```python
from build123d import *

# Parameters (mm, degrees)
F1_DEPTH = 12.7


with BuildPart() as f1:
    # F0 (on Front) → F1 (new body, symmetric)
    with BuildSketch(Plane.XZ):
        Polygon((-41.637809, 68.136583), (-89.650807, -58.443111), (-62.147316, -58.70938), (-31.672317, 17.590671), (0, -58.70938), (90.179723, -58.70938), (75.366612, -24.786401), (48.944038, -24.786401), (52.657543, -33.30938), (15.323475, -33.30938), (-17.810837, 42.736583), (23.85487, 42.736583), (27.09148, 35.308142), (54.189362, 35.308142), (41.60433, 68.136583), align=None)
    extrude(amount=F1_DEPTH, both=True)


solid = f1.part
```
Verification items for the finished model (mm, model axes). A direction names the side the tool comes from. Coordinates: 2 decimals unless noted, no trailing zeros. Loops run counter-clockwise (first coordinate to the right, second up) from the corner with the lowest first, then second, coordinate; pieces in that order, holes last. Notation, with made-up numbers: (72, 15.25) - (114, 15.25) arc R15 cw to (114, 36.25) - close; hole circle Ø10 at (-2.75, 0). An arc over 180 degrees is marked (long way). Return JSON: item names as keys, results as strings.
1. Section check B-B, the plane y = -7. Record the boundary of the cut face in (x, z), then the cut area to 3 significant figures.
Established:
{"outline": "(-89.65, -58.44) - (-62.15, -58.71) - (-31.67, 17.59) - (0, -58.71) - (90.18, -58.71) - (75.37, -24.79) - (48.94, -24.79) - (52.66, -33.31) - (15.32, -33.31) - (-17.81, 42.74) - (23.85, 42.74) - (27.09, 35.31) - (54.19, 35.31) - (41.6, 68.14) - (-41.64, 68.14) - close", "area": "9,620 mm2"}
2. Section check D-D, the plane x = -59. Record the boundary of the cut face in (y, z), then the cut area to 3 significant figures.
Established:
{"outline": "(-12.7, -50.83) - (12.7, -50.83) - (12.7, 22.36) - (-12.7, 22.36) - close", "area": "1,860 mm2"}
3. Mould release check, pull along X, two halves, no side actions. Record for faces 1 (the flat face through (-65.31, -0.18, 5.73)), 2 (the flat face through (-16.058, -0.178, -20.025)), 3 (the flat face through (-1, 12.7, -8)): +X half, -X half, draft (parallel to the pull), parting line (faces both ways), or undercut.
Established:
{"face 1": "-X half", "face 2": "undercut", "face 3": "draft"}
4. Tool access check on faces 4 (the flat face through (50.775, -0.178, -28.988)), 5 (the flat face through (-47.12, -0.18, -21.09)), 6 (the flat face through (62, 0, -24.786)), 7 (the flat face through (1, 0, 68.137)). Record the directions out of +Z, -Z, +X, -X, +Y, -Y that give a thin tool (end or side, any length) a straight path to the whole face; none if there is none.
Established:
{"face 4": "+Y, -Y", "face 5": "-Z, +Y, -Y", "face 6": "+X, +Y, -Y", "face 7": "+Z, +X, -X, +Y, -Y"}
5. Section check C-C, the plane z = 3. Record the boundary of the cut face in (x, y).
Established:
{"outline": "(-66.34, -12.7) - (-37.5, -12.7) - (-37.5, 12.7) - (-66.34, 12.7) - close; (-25.62, -12.7) - (-0.5, -12.7) - (-0.5, 12.7) - (-25.62, 12.7) - close"}
6. Go/stop test with flat-tipped pins: pin 1 (8 mm diameter, centred on y = 2.5, z = -42.5, fed in from +X); pin 2 (2 mm diameter, centred on y = 6.5, z = 53, fed in from +X); pin 3 (2 mm diameter, centred on y = 10, z = 14, fed in from -X). Record where each tip stops, or that it passes through.
Established:
{"pin 1": "stops at x = 84.85", "pin 2": "stops at x = 47.79", "pin 3": "stops at x = -62.55"}
7. Section check A-A, the plane x = 32. Record the boundary of the cut face in (y, z), then the cut area to 3 significant figures.
Established:
{"outline": "(-12.7, -58.71) - (12.7, -58.71) - (12.7, -33.31) - (-12.7, -33.31) - close; (-12.7, 35.31) - (12.7, 35.31) - (12.7, 68.14) - (-12.7, 68.14) - close", "area": "1,480 mm2"}
8. Thickness scan on L1, parallel to X at y = -1.75, z = -32.5; L2, parallel to Z at x = 38, y = 1.5; L3, parallel to X at y = 6.25, z = -21. Record the ranges inside material, lowest first.
Established:
{"L1": "x = -79.81 to -51.68, -10.88 to 14.97, 52.3 to 78.73", "L2": "z = -58.71 to -33.31, 35.31 to 68.14", "L3": "x = -75.45 to -47.09, -15.65 to 9.96"}
